from build123d import *

# Parameters (mm, degrees)
EXTRUDE_1_DEPTH = 45
SKETCH_2_W      = 7
SKETCH_2_H      = 12
EXTRUDE_2_DEPTH = 45


with BuildPart() as part:
    # Эскиз1 → Бобышка-Вытянуть1 (new body)
    with BuildSketch(Plane.XY):
        Polygon((0, 0), (-30, 0), (-30, 30), (-23, 30), (-23, 7), (0, 7), align=None)
    extrude(amount=EXTRUDE_1_DEPTH)

    # Эскиз2 → Бобышка-Вытянуть2 (add)
    with BuildSketch(Plane.XY.offset(45)):
        with Locations((-15.5, -6)):
            Rectangle(SKETCH_2_W, SKETCH_2_H)
    extrude(amount=-EXTRUDE_2_DEPTH)


solid = part.part
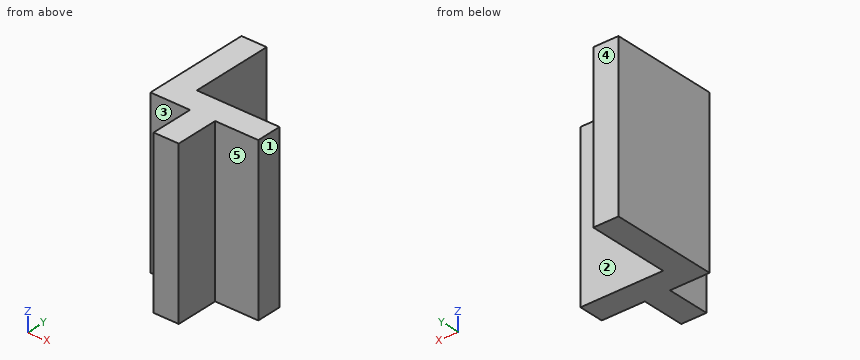
Can you work these out from the model? Positions are in its coordinate system, mm. Face numbers are marked on the shaded views. A direction names the side the tool comes from. Give positions to 0.01 mm unless a question says otherwise; leave off trailing zeros. Write each loop counter-clockwise with the first axis right and the second up, starting at its lowest first coordinate (ties: lowest second). Pieces come first, ordered by that corner, then holes. Notation, with made-up numbers: M 26,41.5 L 76,41.5 A18 cw 76,60.5 Z; hole C 44,44.25 d5. An arc over 180 degrees is marked long. Answer in a Markdown table with one row per item. Add a question column.
Item 1: For pin 1 Ø12 at (y, z) = (16, 11) entering from +X; pin 2 Ø8 at (x, z) = (-20.5, 39.5) entering from -Y; pin 3 Ø3.5 at (x, z) = (-25, 14) entering from -Y; pin 4 Ø1 at (x, z) = (-6, 39) entering from +Y, each with a flat end and sliding along its axis, tell me the tip position at first contact or that it passes through.
Item 2: Imagine slicing it at A-A, the plane z = 8. Write out the boundary of the cut face in (x, y).
Item 3: Please list where these lines run through material, in increasing order: L1, parallel to Y at x = -10, z = 3.5; L2, parallel to X at y = -2, z = 18.5; L3, parallel to X at y = 25.5, z = 12.
Item 4: Imagine slicing it at C-C, the plane y = 9.5. Write out the boundary of the cut face in (x, z).
Item 5: On a 3-axis mill with a long thin cutter (end or side, diameter ignored), from which of +Z, -Z, +X, -X, +Y, -Y can I reach the whole of each face in a straight line? I mean the marked faces 1, 2, 3, 4 and 5. Say none if no direction works.
Item 6: Imagine slicing it at B-B, the plane x = -15.75. Write out the boundary of the cut face in (y, z).
Evaluation:
| question | item | result |
|---|---|---|
| 1 | pin 1 | stops at x = -23 |
| 1 | pin 2 | stops at y = -12 |
| 1 | pin 3 | stops at y = 0 |
| 1 | pin 4 | stops at y = 7 |
| 2 | outline | M -30,0 L -19,0 L -19,-12 L -12,-12 L -12,0 L 0,0 L 0,7 L -23,7 L -23,30 L -30,30 Z |
| 3 | L1 | y = 0 to 7 |
| 3 | L2 | x = -19 to -12 |
| 3 | L3 | x = -30 to -23 |
| 4 | outline | M -30,0 L -23,0 L -23,45 L -30,45 Z |
| 5 | face 1 | +Z, -Z, +X, +Y, -Y |
| 5 | face 2 | +Z, -Z, +X, +Y |
| 5 | face 3 | +Z, -Z, -X, -Y |
| 5 | face 4 | +Z, -Z, +X, -X, +Y |
| 5 | face 5 | +Z, -Z, +X, -Y |
| 6 | outline | M -12,0 L 7,0 L 7,45 L -12,45 Z |
